Build history of the part. All positions in model axes, mm. Face numbers are marked on the shaded views. A direction names the side the tool comes from. Coordinates: 2 decimals unless noted, no trailing zeros. Write each loop counter-clockwise with the first axis right and the second up, starting at its lowest first coordinate (ties: lowest second). Pieces come first, ordered by that corner, then holes.
from build123d import *

# Parameters (mm, degrees)
SKETCH1_W                 = 150
SKETCH1_H                 = 80
BOSS_EXTRUDE1_DEPTH       = 70
SHELL1_T                  = -5
SHELL1_THICKNESS_2_FACE_W = 75
SHELL1_THICKNESS_2_FACE_H = 140
SHELL1_THICKNESS_2_DEPTH  = 15
SKETCH2_W                 = 15
SKETCH2_H                 = 15
FILLET1_R                 = 10


with BuildPart() as part:
    # Sketch1 → Boss-Extrude1 (new body)
    with BuildSketch(Plane(origin=(0, 0, 0), x_dir=(1, 0, 0), z_dir=(0, 1, 0))):
        with Locations((75, 40)):
            Rectangle(SKETCH1_W, SKETCH1_H)
    extrude(amount=BOSS_EXTRUDE1_DEPTH)

    # Shell1
    shell1_openings = [part.faces().sort_by_distance(p)[0] for p in [
        (75, 35, 0),
    ]]
    offset(amount=SHELL1_T, openings=shell1_openings, kind=Kind.INTERSECTION)

    # Shell1 thickness 2 face (on inner face of the shell) → Shell1 thickness 2 (add)
    with BuildSketch(Plane(origin=(75, 65, -37.5), x_dir=(0, 0, 1), z_dir=(0, 1, 0))):
        Rectangle(SHELL1_THICKNESS_2_FACE_W, SHELL1_THICKNESS_2_FACE_H)
    extrude(amount=-SHELL1_THICKNESS_2_DEPTH)

    # Cut-Sweep1: sweep along a path in Sketch3
    with BuildLine(Plane(origin=(0, 70, 0), x_dir=(1, 0, 0), z_dir=(0, 1, 0))) as cut_sweep1_path:
        Line((17.5, 0), (17.5, 65))
        Line((17.5, 65), (54.5, 65))
        Line((54.5, 65), (54.5, 15))
        Line((54.5, 15), (91.5, 15))
        Line((91.5, 15), (91.5, 65))
        Line((91.5, 65), (128.5, 65))
        Line((128.5, 65), (128.5, 15))
    # Sketch2 → Cut-Sweep1 (sweep, cut)
    with BuildSketch(Plane.XY):
        with Locations((17.5, 62.5)):
            Rectangle(SKETCH2_W, SKETCH2_H)
    sweep(path=cut_sweep1_path.line, transition=Transition.RIGHT, mode=Mode.SUBTRACT)

    # Fillet1
    fillet1_edges = [part.edges().sort_by_distance(p)[0] for p in [
        (121, 62.5, -57.5),
        (136, 62.5, -72.5),
        (84, 62.5, -72.5),
        (99, 62.5, -57.5),
        (84, 62.5, -22.5),
        (99, 62.5, -7.5),
        (62, 62.5, -22.5),
        (47, 62.5, -7.5),
        (62, 62.5, -72.5),
        (47, 62.5, -57.5),
        (10, 62.5, -72.5),
        (25, 62.5, -57.5),
    ]]
    fillet(fillet1_edges, radius=FILLET1_R)


solid = part.part
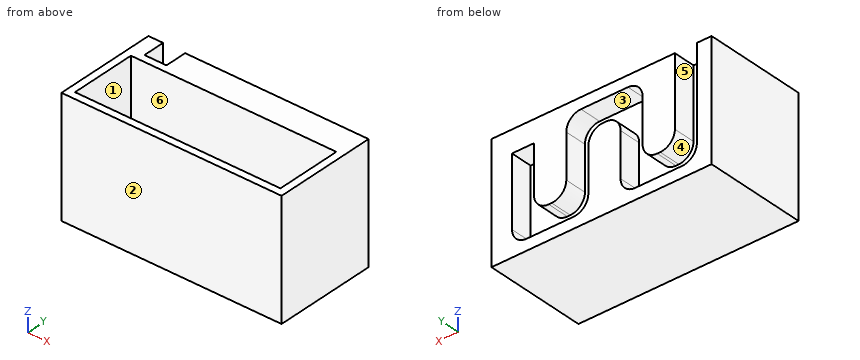
(1) Probe L1, parallel to Y at x = 127, z = -18.5; L2, parallel to Y at x = 81, z = -44; L3, parallel to X at y = 7, z = -45. List the from-to ranges inside material, lowest first.
(2) Slice it at D-D, the plane z = -44.5. List the corners of the cut face in (x, y), and give its area (3 significant figures).
(3) Slice it at A-A, the plane z = -11.5. List the corners of the cut face in (x, y), and give its area (4 significant figures).
(4) Flat gauge pin, fed straight in: P1, Ø13.5, axis at x = 105.5, y = 27, coming from the +Z side. Where does the tip first touch, or does it go through?
(5) Slice it at C-C, the plane x = 82.5. List the corners of the cut face in (y, z).
(6) Slice it at B-B, the plane y = 7. List the corners of the cut face in (x, z), and give its area (3 significant figures).
(7) 3-axis set-ups, long thin cutter, end or side, ignore diameter. For the marked faces 4, 5 and 6: which of +Z, -Z, +X, -X, +Y, -Y reach the whole face in a straight line?
(8) Two-plate mould, pull along Y, no slides. Class the marked faces 1, 2 and 3: pulls with the +Y half, pulls with the -Y half, needs draft (parallel to the pull), parting line crosses it, or undercut.
Results:
1. L1: y = 0 to 5, 50 to 55
1. L2: y = 0 to 5, 50 to 70
1. L3: x = 0 to 5, 145 to 150
2. outline: (0, 0) - (150, 0) - (150, 70) - (136, 70) - (136, 55) - (121, 55) - (121, 70) - (99, 70) - (99, 55) - (84, 55) - (84, 70) - (62, 70) - (62, 55) - (47, 55) - (47, 70) - (25, 70) - (25, 55) - (10, 55) - (10, 70) - (0, 70) - close; hole (5, 5) - (145, 5) - (145, 50) - (5, 50) - close
2. area: 3,300 mm2
3. outline: (0, 0) - (150, 0) - (150, 70) - (97, 70) - (97, 55) - (49, 55) - (49, 70) - (25, 70) - (25, 55) - (10, 55) - (10, 70) - (0, 70) - close; hole (5, 5) - (145, 5) - (145, 50) - (5, 50) - close
3. area: 3,255 mm2
4. P1: stops at z = -75
5. outline: (0, -80) - (70, -80) - (70, -27.23) - (55, -27.23) - (55, -7.5) - (70, -7.5) - (70, 0) - (50, 0) - (50, -75) - (5, -75) - (5, 0) - (0, 0) - close
6. outline: (0, -80) - (150, -80) - (150, 0) - (145, 0) - (145, -75) - (5, -75) - (5, 0) - (0, 0) - close
6. area: 1,500 mm2
7. face 4: +Y
7. face 5: +Z, +Y
7. face 6: +Z
8. face 1: undercut
8. face 2: pulls with the -Y half
8. face 3: needs draft
